Work out the finished part from the listing and answer in its coordinate system (mm). Face numbers are marked on the shaded views. A direction names the side the tool comes from. Give positions to 0.01 mm unless a question says otherwise; leave off trailing zeros. Order: outer loops, then holes, each group sorted by start corner. A loop starts at its lowest first (then second) coordinate and runs counter-clockwise, first axis right, second up. Notation, with made-up numbers: (-18, 57) - (23, 57) arc R24 ccw to (23, 77) - close; hole circle Ø6 at (62, 78). An arc over 180 degrees is marked (long way). Return JSON: item names as keys, results as strings. Group by question number.
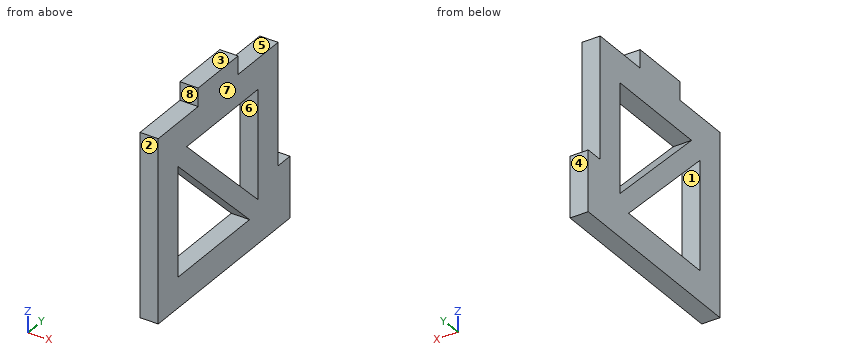
Autodesk Inventor part; units mm, degrees
ref_plane "YZ Plane" through (0, 0, 0) normal (1, 0, 0) x (0, 1, 0)
ref_plane "XZ Plane" through (0, 0, 0) normal (0, 1, 0) x (-1, 0, 0)
ref_plane "XY Plane" through (0, 0, 0) normal (0, 0, 1) x (1, 0, 0)
sketch "Sketch1" plane through (0, 0, 0) normal (1, 0, 0) x (0, 1, 0)
  line L0 (15, -15) -> (-15, -15)
  line L1 (-15, -15) -> (-15, 15)
  line L2 (-15, 15) -> (15, 15)
  line L3 (15, 15) -> (15, -15)
  line L4 (15, -15) -> (-15, 15) construction
  line L5 (-15, -15) -> (15, 15) construction
  line L6 (15, -15) -> (18, -15)
  line L7 (18, -15) -> (18, -5)
  line L8 (18, -5) -> (15, -5)
  line L9 (15, -5) -> (15, -15)
  line L10 (-5, 15) -> (5, 15)
  line L11 (5, 15) -> (5, 18)
  line L12 (5, 18) -> (-5, 18)
  line L13 (-5, 18) -> (-5, 15)
  point P0 (0, 0)
  point P1 (0, 18)
  point P2 (0, 0)
  dimension "d0" = 30
  dimension "d1" = 30
  dimension "d2" = 3
  dimension "d3" = 10
  dimension "d4" = 10
  dimension "d5" = 3
extrude "Extrusion1" add sketch "Sketch1" along normal blind 3
sketch "Sketch2" plane through (0, 0, 0) normal (-1, 0, 0) x (0, 0, 1)
  line L0 (15, -15) -> (-15, -15)
  line L1 (-15, -15) -> (-15, 18)
  line L2 (10, 10) -> (-10, 10)
  line L3 (-10, 10) -> (-10, -10)
  line L4 (-10, -10) -> (10, -10)
  line L5 (10, -10) -> (10, 10)
  line L6 (10, 10) -> (-10, -10) construction
  line L7 (-10, 10) -> (10, -10) construction
  point P0 (0, 0)
  dimension "d8" = 5
  dimension "d9" = 5
extrude "Extrusion2" cut sketch "Sketch2" against normal blind 3
sketch "Sketch3" plane through (0, 0, 0) normal (-1, 0, 0) x (0, 0, 1)
  line L0 (10, -10) -> (-10, -10)
  line L1 (10, 10) -> (10, -10)
  line L2 (-8.9393, 11.0607) -> (11.0607, -8.9393)
  line L3 (11.0607, -8.9393) -> (8.9393, -11.0607)
  line L4 (8.9393, -11.0607) -> (-11.0607, 8.9393)
  line L5 (-11.0607, 8.9393) -> (-8.9393, 11.0607)
  line L6 (-8.9393, 11.0607) -> (8.9393, -11.0607) construction
  line L7 (11.0607, -8.9393) -> (-11.0607, 8.9393) construction
  point P0 (0, 0)
  dimension "d12" = 3
extrude "Extrusion3" add sketch "Sketch3" against normal blind 3
equation "\"d9\" = d8"
properties part number "Motor Side support"
1. Determine the mould class of the marked faces 1, 2 and 3 for opening direction Y: released by +Y, released by -Y, zero draft, split by the parting line, or undercut.
2. The part is cut by section C-C (z = -2). Give the vertices of the cut face in (x, y), and give its area (3 significant figures).
3. The part is cut by section A-A (x = 0.55). Give the vertices of the cut face in (y, z).
4. Consider probe 1 along Z at (x, y) = (2.75, -1); probe 2 along Y at (x, z) = (1.65, 4.5); probe 3 along Z at (x, y) = (1.2, 4). Determine where each line is inside the solid, lowest interval first. Write a range as from..to.
5. The part is cut by section B-B (y = 9.5). Give the vertices of the cut face in (x, z), and give its area (3 significant figures).
6. A tool of negligible diameter and unlimited length cuts with its end or side. For the marked faces 4, 5, 6, 7 and 8, from which of +Z, -Z, +X, -X, +Y, -Y can it reach the whole face along a straight path? Write none if from no direction.
7. The part is cut by section D-D (y = 0.5). Give the vertices of the cut face in (x, z), and give its area (3 significant figures).
8. Each of these flat-tipped pins is pushed along its axis until it touches: pin 1 (1.5 mm diameter, centred on x = 1.5, z = 5, fed in from +Y); pin 2 (1.5 mm diameter, centred on x = 1, y = -8, fed in from +Z). Where does it stop, or does it pass through?
Answers:
{
 "1": {"face 1": "undercut", "face 2": "released by -Y", "face 3": "zero draft"},
 "2": {"outline": "(0, -15) - (3, -15) - (3, -10) - (0, -10) - close; (0, -0.12) - (3, -0.12) - (3, 4.12) - (0, 4.12) - close; (0, 10) - (3, 10) - (3, 15) - (0, 15) - close", "area": "42.7 mm^2"},
 "3": {"outline": "(-15, -15) - (18, -15) - (18, -5) - (15, -5) - (15, 15) - (5, 15) - (5, 18) - (-5, 18) - (-5, 15) - (-15, 15) - close; hole (-10, -10) - (7.88, -10) - (-10, 7.88) - close; hole (-7.88, 10) - (10, -7.88) - (10, 10) - close"},
 "4": {"probe 1": "z = -15..-10, -1.12..3.12, 10..18", "probe 2": "y = -15..-10, -6.62..-2.38, 10..15", "probe 3": "z = -15..-10, -6.12..-1.88, 10..18"},
 "5": {"outline": "(0, -15) - (3, -15) - (3, -7.38) - (0, -7.38) - close; (0, 10) - (3, 10) - (3, 15) - (0, 15) - close", "area": "37.9 mm^2"},
 "6": {"face 4": "+Z, -Z, +X, -X, +Y", "face 5": "+Z, +X, -X, +Y", "face 6": "+X, -X", "face 7": "+Z, -Z, +X, +Y, -Y", "face 8": "+Z, +X, -X, -Y"},
 "7": {"outline": "(0, -15) - (3, -15) - (3, -10) - (0, -10) - close; (0, -2.62) - (3, -2.62) - (3, 1.62) - (0, 1.62) - close; (0, 10) - (3, 10) - (3, 18) - (0, 18) - close", "area": "51.7 mm^2"},
 "8": {"pin 1": "stops at y = 15", "pin 2": "stops at z = 15"}
}
